from build123d import *

# Parameters (mm, degrees)
SKETCH_1_R          = 150
SKETCH_1_R_2        = 2
SKETCH_1_R_3        = 1.75
EXTRUDE_2_DEPTH     = 25
SKETCH_2_R          = 29.5
CUT_EXTRUDE_1_DEPTH = 6.6
SKETCH_3_R          = 50
CUT_EXTRUDE_2_DEPTH = 10
EXTRUDE_START       = 35
SKETCH_10_R         = 150
SKETCH_10_R_2       = 130
EXTRUDE_7_DEPTH     = 35


with BuildPart() as part:
    # 草图1 → 凸台-拉伸2 (new body)
    with BuildSketch(Plane(origin=(0, 0, 0), x_dir=(1, 0, 0), z_dir=(0, 1, 0))):
        with Locations(Location((-17.091633393, 0.301972321, 0), (0, 0, 270))):
            Circle(SKETCH_1_R)
        with Locations(Location((-17.091633393, 17.551972321, 0), (0, 0, 270))):
            Circle(SKETCH_1_R_2, mode=Mode.SUBTRACT)
        with Locations(Location((-17.091633393, 42.801972321, 0), (0, 0, 270))):
            Circle(SKETCH_1_R_3, mode=Mode.SUBTRACT)
        with Locations(Location((12.960404807, 30.354010522, 0), (0, 0, 270))):
            Circle(SKETCH_1_R_3, mode=Mode.SUBTRACT)
        with Locations(Location((25.408366607, 0.301972321, 0), (0, 0, 270))):
            Circle(SKETCH_1_R_3, mode=Mode.SUBTRACT)
        with Locations(Location((12.960404807, -29.750065879, 0), (0, 0, 270))):
            Circle(SKETCH_1_R_3, mode=Mode.SUBTRACT)
        with Locations(Location((-17.091633393, -42.198027679, 0), (0, 0, 270))):
            Circle(SKETCH_1_R_3, mode=Mode.SUBTRACT)
        with Locations(Location((-47.143671594, -29.750065879, 0), (0, 0, 270))):
            Circle(SKETCH_1_R_3, mode=Mode.SUBTRACT)
        with Locations(Location((-59.591633393, 0.301972321, 0), (0, 0, 270))):
            Circle(SKETCH_1_R_3, mode=Mode.SUBTRACT)
        with Locations(Location((-47.143671594, 30.354010522, 0), (0, 0, 270))):
            Circle(SKETCH_1_R_3, mode=Mode.SUBTRACT)
        with Locations(Location((-2.152695178, 8.926972321, 0), (0, 0, 270))):
            Circle(SKETCH_1_R_2, mode=Mode.SUBTRACT)
        with Locations(Location((-2.152695178, -8.323027679, 0), (0, 0, 270))):
            Circle(SKETCH_1_R_2, mode=Mode.SUBTRACT)
        with Locations(Location((-17.091633393, -16.948027679, 0), (0, 0, 270))):
            Circle(SKETCH_1_R_2, mode=Mode.SUBTRACT)
        with Locations(Location((-32.030571609, -8.323027679, 0), (0, 0, 270))):
            Circle(SKETCH_1_R_2, mode=Mode.SUBTRACT)
        with Locations(Location((-32.030571609, 8.926972321, 0), (0, 0, 270))):
            Circle(SKETCH_1_R_2, mode=Mode.SUBTRACT)
    extrude(amount=EXTRUDE_2_DEPTH)

    # 草图2 → 切除-拉伸1 (cut)
    with BuildSketch(Plane.XZ):
        with Locations(Location((-17.091633393, -0.301972321, 0), (0, 0, 270))):
            Circle(SKETCH_2_R)
    extrude(amount=-CUT_EXTRUDE_1_DEPTH, mode=Mode.SUBTRACT)

    # 草图3 → 切除-拉伸2 (cut)
    with BuildSketch(Plane(origin=(0, 25, 0), x_dir=(1, 0, 0), z_dir=(0, 1, 0))):
        with Locations(Location((-16.888033671, 0.912771488, 0), (0, 0, 270))):
            Circle(SKETCH_3_R)
    extrude(amount=-CUT_EXTRUDE_2_DEPTH, mode=Mode.SUBTRACT)

    # 草图10 → 凸台-拉伸7 (add)
    with BuildSketch(Plane.XZ.offset(EXTRUDE_START)):
        with Locations(Location((-17.091633393, -0.301972321, 0), (0, 0, 270))):
            Circle(SKETCH_10_R)
        with Locations(Location((-17.091633393, -0.301972321, 0), (0, 0, 270))):
            Circle(SKETCH_10_R_2, mode=Mode.SUBTRACT)
    extrude(amount=-EXTRUDE_7_DEPTH)


solid = part.part
For this review, take the finished solid that the model builds, in its own axes (mm). A direction names the side the tool comes from. Give positions to 0.01 mm unless a question says otherwise; leave off trailing zeros. Order: outer loops, then holes, each group sorted by start corner. A loop starts at its lowest first (then second) coordinate and runs counter-clockwise, first axis right, second up. Notation, with made-up numbers: (60.5, 44.5) -> (115.5, 44.5) arc R26 ccw to (115.5, 71.5) -> close; hole circle Ø1 at (32, 18). An arc over 180 degrees is marked (long way). Write item = value, one per line.
1) For faces 3 (the face through (-16, 15, -2)), 4 (the face through (-82, 25, -2)), 5 (the face through (12.157, 3.254, 3.538)), list the 3-axis set-ups (+Z, -Z, +X, -X, +Y, -Y) from which the entire face can be reached by the end or side of a thin tool; tool diameter is ignored.
Findings:
face_3 = +Y
face_4 = +Z, -Z, +X, -X, +Y
face_5 = -Y
2) We need section D-D, the plane y = -5.5. Give the boundary of the cut face in (x, z).
Findings:
outline = circle Ø300 at (-17.09, -0.3); hole circle Ø260 at (-17.09, -0.3)
3) We need section B-B, the plane y = 10.5. Count the separate pieces of the cut face and the enclosed holes in it, and give its area (3 significant figures).
Findings:
separate_pieces = 1
enclosed_holes = 14
area = 70,500 mm^2
4) Draft analysis for pull direction Z (two halves, no side actions). For faces 1 (the face through (14, 0, -2)), 2 (the face through (106, -35, 45)), state which applies: pulls with the +Z half, pulls with the -Z half, needs draft (parallel to the pull), parting line crosses it, or undercut.
Findings:
face_1 = undercut
face_2 = needs draft
5) Insertion check: pin 1 (6 mm diameter, centred on x = -67.5, z = -98.5, fed in from -Y); pin 2 (1 mm diameter, centred on y = -17.5, z = 42, fed in from -X); pin 3 (8 mm diameter, centred on y = -24.5, z = -75.5, fed in from +X). Each pin has a flat end and moves straight along its axis. Give the tip position at first contact, or say it passes through.
Findings:
pin_1 = 0
pin_2 = -161.15
pin_3 = 114.93
6) We need section A-A, the plane x = -110. Give the boundary of the cut face in (y, z).
Findings:
outline = (-35, -118.06) -> (25, -118.06) -> (25, 117.46) -> (-35, 117.46) -> (-35, 90.63) -> (0, 90.63) -> (0, -91.23) -> (-35, -91.23) -> close
7) To check wall thickness, follow L1, parallel to Z at x = -20, y = -2; L2, parallel to Z at x = -63, y = -1.5; L3, parallel to X at y = 16, z = 29. State the ranges of each line that lie inside material, in increasing order. Write a range as from..to.
Findings:
L1 = -150.27..-130.27, 129.67..149.67
L2 = -143.1..-121.93, 121.32..142.5
L3 = -164.2..-56.95, 23.18..130.02
8) We need section C-C, the plane z = -102.5. Give the boundary of the cut face in (x, y), and give its area (3 significant figures).
Findings:
outline = (-126.89, -35) -> (-97.44, -35) -> (-97.44, 0) -> (63.25, 0) -> (63.25, -35) -> (92.71, -35) -> (92.71, 25) -> (-126.89, 25) -> close
area = 7,550 mm^2
